```python
from build123d import *
from build123d.topology import SkipClean

# Parameters (mm, degrees)
CROQUIS1_W                  = 130.4
CROQUIS1_H                  = 60
SALIENTE_EXTRUIR1_DEPTH     = 2
CROQUIS3_W                  = 65.2
CROQUIS3_H                  = 12.2
CROQUIS3_R                  = 1
SALIENTE_EXTRUIR2_DEPTH     = 2
CORTAR_EXTRUIR2_REACH       = 91.737
CROQUIS5_W                  = 24
CROQUIS5_H                  = 12.2
CROQUIS6_W                  = 4.675
CROQUIS6_H                  = 5
CROQUIS6_R                  = 1.375
CROQUIS6_W_2                = 9.35
SALIENTE_EXTRUIR3_DEPTH     = 12.2
SIMETR_A2_COPY_1_SKETCH_W   = 65.2
SIMETR_A2_COPY_1_SKETCH_H   = 12.2
SIMETR_A2_COPY_1_SKETCH_R   = 1
SIMETR_A2_COPY_1_DEPTH      = 2
SIMETR_A2_COPY_2_REACH      = 91.737
SIMETR_A2_COPY_2_SKETCH_W   = 24
SIMETR_A2_COPY_2_SKETCH_H   = 12.2
SIMETR_A2_COPY_3_SKETCH_W   = 4.675
SIMETR_A2_COPY_3_SKETCH_H   = 5
SIMETR_A2_COPY_3_SKETCH_R   = 1.375
SIMETR_A2_COPY_3_SKETCH_W_2 = 9.35
SIMETR_A2_COPY_3_DEPTH      = 12.2
CHAFL_N1_SIZE               = 1
CROQUIS7_W                  = 2
CROQUIS7_H                  = 42.8
SALIENTE_EXTRUIR4_DEPTH     = 12.2
CHAFL_N2_SIZE               = 1
CROQUIS9_W                  = 70
CROQUIS9_H                  = 18
CORTAR_EXTRUIR4_DEPTH       = 12


with BuildPart() as part:
    # Croquis1 → Saliente-Extruir1 (new body)
    with BuildSketch(Plane(origin=(0, 0, 0), x_dir=(1, 0, 0), z_dir=(0, 1, 0))):
        Rectangle(CROQUIS1_W, CROQUIS1_H)
    extrude(amount=SALIENTE_EXTRUIR1_DEPTH)

    # Croquis3 → Saliente-Extruir2 (add)
    with BuildSketch(Plane.XY.offset(30)):
        with Locations((-32.6, 8.1)):
            Rectangle(CROQUIS3_W, CROQUIS3_H)
        with Locations((-62.85, 8.1)):
            Circle(CROQUIS3_R, mode=Mode.SUBTRACT)
        with Locations((-34.95, 8.1)):
            Circle(CROQUIS3_R, mode=Mode.SUBTRACT)
        with Locations(Location((-30.25, 8.1, 0), (0, 0, 180))):
            Circle(CROQUIS3_R, mode=Mode.SUBTRACT)
        with Locations(Location((-2.35, 8.1, 0), (0, 0, 180))):
            Circle(CROQUIS3_R, mode=Mode.SUBTRACT)
    saliente_extruir2 = extrude(amount=-SALIENTE_EXTRUIR2_DEPTH)

    # Croquis5 → Cortar-Extruir2 (cut, up to next)
    with BuildSketch(Plane.XY.offset(30), mode=Mode.PRIVATE) as cortar_extruir2_sk1:
        with Locations((-48.9, 8.1)):
            Rectangle(CROQUIS5_W, CROQUIS5_H)
    cortar_extruir2_tool1 = extrude(cortar_extruir2_sk1.sketch, amount=-CORTAR_EXTRUIR2_REACH, mode=Mode.PRIVATE) & part.part
    # Croquis5 → Cortar-Extruir2 (cut, up to next)
    with BuildSketch(Plane.XY.offset(30), mode=Mode.PRIVATE) as cortar_extruir2_sk2:
        with Locations((-16.3, 8.1)):
            Rectangle(CROQUIS5_W, CROQUIS5_H)
    cortar_extruir2_tool2 = extrude(cortar_extruir2_sk2.sketch, amount=-CORTAR_EXTRUIR2_REACH, mode=Mode.PRIVATE) & part.part
    cortar_extruir2_1 = cortar_extruir2_tool1.solids().sort_by_distance((-48.9, 8.1, 30))[0]
    add(cortar_extruir2_1, mode=Mode.SUBTRACT)
    cortar_extruir2_2 = cortar_extruir2_tool2.solids().sort_by_distance((-16.3, 8.1, 30))[0]
    add(cortar_extruir2_2, mode=Mode.SUBTRACT)
    cortar_extruir2 = cortar_extruir2_1 + cortar_extruir2_2  # Cortar-Extruir2 as one shape, for the pattern or mirror that repeats it

    # Croquis6 → Saliente-Extruir3 (add)
    # profile 1 of 3: a face of its own
    with BuildSketch(Plane(origin=(0, 2, 0), x_dir=(1, 0, 0), z_dir=(0, 1, 0))):
        with Locations((-62.8625, -23.9)):
            Rectangle(CROQUIS6_W, CROQUIS6_H)
        with Locations(Location((-62.856394864, -23.9, 0), (0, 0, 270))):
            Circle(CROQUIS6_R, mode=Mode.SUBTRACT)
    # profile 2 of 3: a face of its own
    with BuildSketch(Plane(origin=(0, 2, 0), x_dir=(1, 0, 0), z_dir=(0, 1, 0))):
        with Locations((-32.6, -23.9)):
            Rectangle(CROQUIS6_W_2, CROQUIS6_H)
        with Locations(Location((-32.6, -23.9, 0), (0, 0, 270))):
            Circle(CROQUIS6_R, mode=Mode.SUBTRACT)
    # profile 3 of 3: a face of its own
    with BuildSketch(Plane(origin=(0, 2, 0), x_dir=(1, 0, 0), z_dir=(0, 1, 0))):
        with BuildLine():
            Line((-4.675, -21.4), (0, -21.4))
            Line((0, -21.4), (0, -22.525))
            ThreePointArc((0, -22.525), (-1.375, -23.9), (0, -25.275))
            Line((0, -25.275), (0, -26.4))
            Line((0, -26.4), (-4.675, -26.4))
            Line((-4.675, -26.4), (-4.675, -21.4))
        make_face()
    saliente_extruir3 = extrude(amount=SALIENTE_EXTRUIR3_DEPTH)

    # Simetría1: Saliente-Extruir2, Cortar-Extruir2, Saliente-Extruir3 across plane
    add(saliente_extruir2.mirror(Plane(origin=(0, 0, 0), x_dir=(0, 0, 1), z_dir=(1, 0, 0))))
    add(cortar_extruir2.mirror(Plane(origin=(0, 0, 0), x_dir=(0, 0, 1), z_dir=(1, 0, 0))), mode=Mode.SUBTRACT)
    add(saliente_extruir3.mirror(Plane(origin=(0, 0, 0), x_dir=(0, 0, 1), z_dir=(1, 0, 0))))

    # Simetría2: Saliente-Extruir2, Cortar-Extruir2, Saliente-Extruir3 across plane
    add(saliente_extruir2.mirror(Plane.XY))
    add(cortar_extruir2.mirror(Plane.XY), mode=Mode.SUBTRACT)
    add(saliente_extruir3.mirror(Plane.XY))

    # Simetría2 copy 1 sketch → Simetría2 copy 1 (add)
    with BuildSketch(Plane(origin=(0, 0, -30), x_dir=(-1, 0, 0), z_dir=(0, 0, -1))):
        with Locations((-32.6, 8.1)):
            Rectangle(SIMETR_A2_COPY_1_SKETCH_W, SIMETR_A2_COPY_1_SKETCH_H)
        with Locations((-62.85, 8.1)):
            Circle(SIMETR_A2_COPY_1_SKETCH_R, mode=Mode.SUBTRACT)
        with Locations((-34.95, 8.1)):
            Circle(SIMETR_A2_COPY_1_SKETCH_R, mode=Mode.SUBTRACT)
        with Locations(Location((-30.25, 8.1, 0), (0, 0, 180))):
            Circle(SIMETR_A2_COPY_1_SKETCH_R, mode=Mode.SUBTRACT)
        with Locations(Location((-2.35, 8.1, 0), (0, 0, 180))):
            Circle(SIMETR_A2_COPY_1_SKETCH_R, mode=Mode.SUBTRACT)
    extrude(amount=-SIMETR_A2_COPY_1_DEPTH)

    # Simetría2 copy 2 sketch → Simetría2 copy 2 (cut, up to next)
    with BuildSketch(Plane(origin=(0, 0, -30), x_dir=(-1, 0, 0), z_dir=(0, 0, -1)), mode=Mode.PRIVATE) as simetr_a2_copy_2_sk1:
        with Locations((-48.9, 8.1)):
            Rectangle(SIMETR_A2_COPY_2_SKETCH_W, SIMETR_A2_COPY_2_SKETCH_H)
    simetr_a2_copy_2_tool1 = extrude(simetr_a2_copy_2_sk1.sketch, amount=-SIMETR_A2_COPY_2_REACH, mode=Mode.PRIVATE) & part.part
    # Simetría2 copy 2 sketch → Simetría2 copy 2 (cut, up to next)
    with BuildSketch(Plane(origin=(0, 0, -30), x_dir=(-1, 0, 0), z_dir=(0, 0, -1)), mode=Mode.PRIVATE) as simetr_a2_copy_2_sk2:
        with Locations((-16.3, 8.1)):
            Rectangle(SIMETR_A2_COPY_2_SKETCH_W, SIMETR_A2_COPY_2_SKETCH_H)
    simetr_a2_copy_2_tool2 = extrude(simetr_a2_copy_2_sk2.sketch, amount=-SIMETR_A2_COPY_2_REACH, mode=Mode.PRIVATE) & part.part
    add(simetr_a2_copy_2_tool1.solids().sort_by_distance((48.9, 8.1, -30))[0], mode=Mode.SUBTRACT)
    add(simetr_a2_copy_2_tool2.solids().sort_by_distance((16.3, 8.1, -30))[0], mode=Mode.SUBTRACT)

    # Simetría2 copy 3 sketch → Simetría2 copy 3 (add)
    # profile 1 of 3: a face of its own
    with SkipClean():  # the faces are left unmerged after this step: merging them gives an invalid solid
        with BuildSketch(Plane(origin=(0, 2, 0), x_dir=(-1, 0, 0), z_dir=(0, 1, 0))):
            with Locations((-62.8625, -23.9)):
                Rectangle(SIMETR_A2_COPY_3_SKETCH_W, SIMETR_A2_COPY_3_SKETCH_H)
            with Locations(Location((-62.856394864, -23.9, 0), (0, 0, 270))):
                Circle(SIMETR_A2_COPY_3_SKETCH_R, mode=Mode.SUBTRACT)
        # profile 2 of 3: a face of its own
        with BuildSketch(Plane(origin=(0, 2, 0), x_dir=(-1, 0, 0), z_dir=(0, 1, 0))):
            with Locations((-32.6, -23.9)):
                Rectangle(SIMETR_A2_COPY_3_SKETCH_W_2, SIMETR_A2_COPY_3_SKETCH_H)
            with Locations(Location((-32.6, -23.9, 0), (0, 0, 270))):
                Circle(SIMETR_A2_COPY_3_SKETCH_R, mode=Mode.SUBTRACT)
        # profile 3 of 3: a face of its own
        with BuildSketch(Plane(origin=(0, 2, 0), x_dir=(-1, 0, 0), z_dir=(0, 1, 0))):
            with BuildLine():
                Line((-4.675, -21.4), (0, -21.4))
                Line((0, -21.4), (0, -22.525))
                ThreePointArc((0, -22.525), (-1.375, -23.9), (0, -25.275))
                Line((0, -25.275), (0, -26.4))
                Line((0, -26.4), (-4.675, -26.4))
                Line((-4.675, -26.4), (-4.675, -21.4))
            make_face()
        extrude(amount=SIMETR_A2_COPY_3_DEPTH)

    # Chaflán1
    chafl_n1_edges = [part.edges().sort_by_distance(p)[0] for p in [
        (0, 0, 30),
        (-65.2, 0, 0),
        (0, 0, -30),
        (65.2, 0, 0),
    ]]
    chamfer(chafl_n1_edges, length=CHAFL_N1_SIZE)

    # Croquis7 → Saliente-Extruir4 (add)
    with SkipClean():  # the faces are left unmerged after this step: merging them gives an invalid solid
        with BuildSketch(Plane(origin=(0, 2, 0), x_dir=(1, 0, 0), z_dir=(0, 1, 0))):
            with Locations((-32.6, 0)):
                Rectangle(CROQUIS7_W, CROQUIS7_H)
            with Locations((32.6, 0)):
                Rectangle(CROQUIS7_W, CROQUIS7_H)
        extrude(amount=SALIENTE_EXTRUIR4_DEPTH)

    # Chaflán2
    chafl_n2_edges = [part.edges().sort_by_distance(p)[0] for p in [
        (0, 2, 21.4),
        (62.8625, 2, 21.4),
        (29.7625, 2, 21.4),
        (62.8625, 2, -21.4),
        (29.7625, 2, -21.4),
        (-2.3375, 2, -21.4),
        (-62.8625, 2, -21.4),
        (-29.7625, 2, -21.4),
        (-35.4375, 2, -21.4),
        (-35.4375, 2, 21.4),
        (-31.6, 2, 0),
        (-33.6, 2, 0),
        (35.4375, 2, -21.4),
        (35.4375, 2, 21.4),
        (33.6, 2, 0),
        (31.6, 2, 0),
        (-62.8625, 2, 21.4),
    ]]
    chamfer(chafl_n2_edges, length=CHAFL_N2_SIZE)

    # Croquis9 → Cortar-Extruir4 (cut)
    with SkipClean():  # the faces are left unmerged after this step: merging them gives an invalid solid
        with BuildSketch(Plane.XZ):
            Rectangle(CROQUIS9_W, CROQUIS9_H)
        extrude(amount=-CORTAR_EXTRUIR4_DEPTH, mode=Mode.SUBTRACT)


solid = part.part
```
Geometry: final body of the model. Coordinates: model frame, mm. A direction names the side the tool comes from. Round coordinates to 2 decimals unless told otherwise and drop trailing zeros. Write each loop counter-clockwise with the first axis right and the second up, starting at its lowest first coordinate (ties: lowest second). Pieces come first, ordered by that corner, then holes. Notation, with made-up numbers: (6, -18) -> (19, -18) arc R18 ccw to (19, 3) -> close; hole circle Ø8 at (63.5, -21). An arc over 180 degrees is marked (long way). Use CSV: the item, a comma, the result in double quotes. Start each with the question number.
Q1. Pull-direction query (Z, two-part tool) for faces 6 (the face through (-64.08, 8.01, -24.53)), 7 (the face through (-27.925, 8, -24)), 8 (the face through (5, 1.5, -9)); classes: pulls with the +Z half, pulls with the -Z half, needs draft (parallel to the pull), parting line crosses it, or undercut.
Q2. Reachability of faces 1 (the face through (-35, 9, -21.4)), 2 (the face through (33, 8, 26.4)), 3 (the face through (-27.925, 8, 24)), 4 (the face through (-33, 2, -24)), 5 (the face through (33.6, 12.3, 0.3)) from +Z, -Z, +X, -X, +Y, -Y: full face, straight path, thin tool, end or side. Return the list, or none.
Q3. Section B-B (x = -38.5). Return loops of the section in (y, z).
Q4. Section C-C (y = 5.75). Give the number of separate pieces and of enclosed holes in the cut face, plus the area to 3 significant figures.
Q5. First-contact query: pin 1 Ø1.2 at (x, y) = (30.25, 8.1) entering from +Z; pin 2 Ø2 at (y, z) = (7.5, -17) entering from +X; pin 3 Ø4.5 at (x, z) = (62.86, -23.9) entering from +Y; pin 4 Ø1.1 at (x, y) = (-30.5, 8) entering from -Z. Flat tips, straight axial feed; report the tip coordinate or a pass-through.
Q6. Section A-A (z = 0). Return loops of the section in (x, y), plus the area to 3 significant figures.
Q7. Line query: L1, parallel to Z at x = -30, y = 12.25; L2, parallel to X at y = 4.5, z = -21.5 (3 decimals); L3, parallel to Z at x = 32.6, y = 7.75 (3 decimals). Output: solid intervals per line, ascending.
Result sheet:
1,face 6,"undercut"
1,face 7,"needs draft"
1,face 8,"undercut"
2,face 1,"-X, +Y"
2,face 2,"+X, -X, +Y"
2,face 3,"+Z, -Z, +Y"
2,face 4,"+Y"
2,face 5,"+X, +Y"
3,outline,"(0, -29) -> (1, -30) -> (2, -30) -> (2, 30) -> (1, 30) -> (0, 29) -> close"
4,separate pieces,"20"
4,enclosed holes,"10"
4,area,"551 mm²"
5,pin 1,"z = 26.4"
5,pin 2,"x = 33.6"
5,pin 3,"y = 14.2"
5,pin 4,"z = -26.4"
6,outline,"(-65.2, 1) -> (-64.2, 0) -> (-35, 0) -> (-35, 2) -> (-65.2, 2) -> close; (-33.6, 12) -> (-31.6, 12) -> (-31.6, 14.2) -> (-33.6, 14.2) -> close; (31.6, 12) -> (33.6, 12) -> (33.6, 14.2) -> (31.6, 14.2) -> close; (35, 0) -> (64.2, 0) -> (65.2, 1) -> (65.2, 2) -> (35, 2) -> close"
6,area,"129 mm²"
7,L1,"-30 to -28, -26.4 to -21.4, 21.4 to 26.4, 28 to 30"
7,L2,"-65.2 to -60.525, -37.275 to -27.925, -4.675 to 4.675, 27.925 to 37.275, 60.525 to 65.2"
7,L3,"-30 to -28, -26.4 to -25.275, -22.525 to -9, 9 to 22.525, 25.275 to 26.4, 28 to 30"
